The listing builds one solid part. Answer for the finished solid, in the listing's coordinates (mm). A direction names the side the tool comes from. Round coordinates to 2 decimals unless told otherwise and drop trailing zeros. Order: outer loops, then holes, each group sorted by start corner. A loop starts at its lowest first (then second) coordinate and runs counter-clockwise, first axis right, second up. Notation, with made-up numbers: (-29.5, 74) - (-6.5, 74) arc R6 cw to (-6.5, 84) - close; hole circle Ø7 at (-19.5, 35). An arc over 180 degrees is marked (long way). One line per item, written item: value. Start each with the question number.
1. For a pull along Y with two mould halves and no side action, classify faces 5 (the flat face through (-60, -9.941, 57)), 6 (the flat face through (-72.639, -2, -16)), 7 (the flat face through (-32, 19.559, -5)), 8 (the flat face through (-57, 5.559, -21)) as released by +Y, released by -Y, zero draft, split by the parting line, or undercut.
2. Section B-B, the plane x = -48 is taken. Give the vertices of the cut face in (y, z), then the cut area to 3 significant figures.
3. Section D-D, the plane x = -6.5 is taken. Give the vertices of the cut face in (y, z).
4. Section A-A, the plane z = -25 is taken. Give the vertices of the cut face in (x, y).
5. Flat-ended cylindrical pins translate along their axes: P1, Ø12, axis at x = 7.5, y = 18, coming from the -Z side; P2, Ø11, axis at x = -58.5, z = 88, coming from the -Y side; P3, Ø4, axis at y = 10, z = 30.5, coming from the +X side; P4, Ø11, axis at x = -58.5, z = 41, coming from the +Y side. Find the tip coordinate at first contact, or state that the pin passes through.
6. Straight lines are drawn through the part: line 1 (X direction, y = -0.5, z = -25); line 2 (Z direction, x = -21.5, y = 20); line 3 (X direction, y = -7, z = 59). For each, find the intervals that lie inside material, in ascending order.
7. A tool of negligible diameter and unlimited length cuts with its end or side. For faces 1 (the flat face through (-28.113, 13.002, -5.07)), 2 (the flat face through (-42.639, -2, -25)), 3 (the flat face through (-60, 4, 104.21)), 4 (the flat face through (-55.139, -9, 57)), from which of +Z, -Z, +X, -X, +Y, -Y can it reach the whole face along a straight path? Write none if from no direction.
8. Section C-C, the plane z = 96 is taken. Give the vertices of the cut face in (x, y).
from build123d import *

# Parameters (mm, degrees)
SKETCH3_W             = 42.5
SKETCH3_H             = 15
BOSS_EXTRUDE1_DEPTH   = 10
CUT_EXTRUDE1_DEPTH    = 2.5
SKETCH11_W            = 42.5
SKETCH11_H            = 10
BOSS_EXTRUDE5_DEPTH   = 10
SKETCH14_W            = 42.5
SKETCH14_H            = 10
BOSS_EXTRUDE7_DEPTH   = 15
SKETCH20_W            = 10
SKETCH20_H            = 40
BOSS_EXTRUDE10_DEPTH  = 50
SKETCH21_W            = 10
SKETCH21_H            = 25
BOSS_EXTRUDE11_DEPTH  = 113.5
SKETCH22_W            = 30
SKETCH22_H            = 6
BOSS_EXTRUDE12_DEPTH  = 30
SKETCH23_W            = 30
SKETCH23_H            = 30
BOSS_EXTRUDE13_DEPTH  = 8.5
FILLET1_R             = 3
CHAMFER1_SIZE         = 15
CHAMFER1_SIZE2        = 30.41699103
FILLET2_R             = 3
CHAMFER2_SIZE         = 10
CHAMFER2_SIZE2        = 17.320508076
FILLET3_R             = 5
CUT_EXTRUDE2_DEPTH    = 144.583262507
FILLET4_R             = 3
FILLET5_R             = 1.5
M8_TAPPED_HOLE1_D     = 6.8
M8_TAPPED_HOLE1_DEPTH = 22.25
M8_TAPPED_HOLE1_TIP   = 2.042926105
CUT_EXTRUDE3_DEPTH    = 141.312152004
FILLET6_R             = 1.5


with BuildPart() as part:
    # Sketch3 → Boss-Extrude1 (new body)
    with BuildSketch(Plane.XY):
        with Locations((-1.388845539, 0.05888455)):
            Rectangle(SKETCH3_W, SKETCH3_H)
    extrude(amount=-BOSS_EXTRUDE1_DEPTH)

    # Sketch2 → Cut-Extrude1 (cut)
    with BuildSketch(Plane.XY):
        with BuildLine():
            Line((-16.888114198, 2.469689731), (-3.968626967, 4.5))
            ThreePointArc((-3.968626967, 4.5), (0, 6), (3.968626967, 4.5))
            Line((3.968626967, 4.5), (16.888114198, 2.469689731))
            ThreePointArc((16.888114198, 2.469689731), (19, 0), (16.888114198, -2.469689731))
            Line((16.888114198, -2.469689731), (3.968626967, -4.5))
            ThreePointArc((3.968626967, -4.5), (0, -6), (-3.968626967, -4.5))
            Line((-3.968626967, -4.5), (-16.888114198, -2.469689731))
            ThreePointArc((-16.888114198, -2.469689731), (-19, 0), (-16.888114198, 2.469689731))
        make_face()
    extrude(amount=-CUT_EXTRUDE1_DEPTH, mode=Mode.SUBTRACT)

    # Sketch11 → Boss-Extrude5 (add)
    with BuildSketch(Plane.XZ.offset(7.44111545)):
        with Locations((-1.388845539, -5)):
            Rectangle(SKETCH11_W, SKETCH11_H)
    extrude(amount=BOSS_EXTRUDE5_DEPTH)

    # Sketch14 → Boss-Extrude7 (add)
    with BuildSketch(Plane(origin=(0, 7.55888455, 0), x_dir=(1, 0, 0), z_dir=(0, 1, 0))):
        with Locations((-1.388845539, 5)):
            Rectangle(SKETCH14_W, SKETCH14_H)
    extrude(amount=BOSS_EXTRUDE7_DEPTH)

    # Sketch20 → Boss-Extrude10 (add)
    with BuildSketch(Plane.ZY.offset(22.638845539)):
        with Locations((-5, 2.55888455)):
            Rectangle(SKETCH20_W, SKETCH20_H)
    extrude(amount=BOSS_EXTRUDE10_DEPTH)

    # Sketch21 → Boss-Extrude11 (add)
    with BuildSketch(Plane.XY):
        with Locations((-60.138845539, 2.55888455)):
            Rectangle(SKETCH21_W, SKETCH21_H)
    extrude(amount=BOSS_EXTRUDE11_DEPTH)

    # Sketch22 → Boss-Extrude12 (add)
    with BuildSketch(Plane(origin=(0, 0, -10), x_dir=(-1, 0, 0), z_dir=(0, 0, -1))):
        with Locations((57.638845539, 2.55888455)):
            Rectangle(SKETCH22_W, SKETCH22_H)
    extrude(amount=BOSS_EXTRUDE12_DEPTH)

    # Sketch23 → Boss-Extrude13 (add)
    with BuildSketch(Plane.XZ.offset(0.44111545)):
        with Locations((-57.638845539, -25)):
            Rectangle(SKETCH23_W, SKETCH23_H)
    extrude(amount=BOSS_EXTRUDE13_DEPTH)

    # Fillet1
    fillet1_edges = [part.edges().sort_by_distance(p)[0] for p in [
        (-65.138845539, 2.55888455, 0),
        (-60.138845539, -9.94111545, 0),
        (-55.138845539, 2.55888455, 0),
        (-60.138845539, 15.05888455, 0),
    ]]
    fillet(fillet1_edges, radius=FILLET1_R)

    # Chamfer1
    chamfer1_edges = [part.edges().sort_by_distance(p)[0] for p in [
        (19.861154461, 22.55888455, -5),
    ]]
    chamfer1_side = [part.faces().sort_by_distance(p)[0] for p in [
        (19.861154461, 2.55888455, -5),
    ]]
    chamfer(chamfer1_edges, length=CHAMFER1_SIZE, length2=CHAMFER1_SIZE2, reference=chamfer1_side[0])

    # Fillet2
    fillet2_edges = [part.edges().sort_by_distance(p)[0] for p in [
        (-10.555836569, 22.55888455, -5),
        (19.861154461, 7.55888455, -5),
    ]]
    fillet(fillet2_edges, radius=FILLET2_R)

    # Chamfer2
    chamfer2_edges = [part.edges().sort_by_distance(p)[0] for p in [
        (19.861154461, -17.44111545, -5),
    ]]
    chamfer2_side = [part.faces().sort_by_distance(p)[0] for p in [
        (19.861154461, -5.873875391, -5),
    ]]
    chamfer(chamfer2_edges, length=CHAMFER2_SIZE, length2=CHAMFER2_SIZE2, reference=chamfer2_side[0])

    # Fillet3
    fillet3_edges = [part.edges().sort_by_distance(p)[0] for p in [
        (2.540646385, -17.44111545, -5),
        (19.861154461, -7.44111545, -5),
    ]]
    fillet(fillet3_edges, radius=FILLET3_R)

    # Sketch24 → Cut-Extrude2 (cut, through all)
    with BuildSketch(Plane.ZY.offset(65.138845539)):
        Polygon((58.25, -6.94111545), (95.25, -6.94111545), (58.25, 12.05888455), (21.25, -6.94111545), align=None)
        Polygon((48.39896268, 12.05888455), (12.290027833, -6.483541453), (12.290027833, 12.05888455), align=None)
        Polygon((68.10103732, 12.05888455), (104.209972167, 12.05888455), (104.209972167, -6.483541453), align=None)
    extrude(amount=-CUT_EXTRUDE2_DEPTH, mode=Mode.SUBTRACT)

    # Fillet4
    fillet4_edges = [part.edges().sort_by_distance(p)[0] for p in [
        (-60.138845539, -6.483541453, 104.209972167),
        (-60.138845539, 12.05888455, 104.209972167),
        (-60.138845539, 12.05888455, 12.290027833),
        (-60.138845539, -6.483541453, 12.290027833),
        (-60.138845539, 12.05888455, 58.25),
    ]]
    fillet(fillet4_edges, radius=FILLET4_R)

    # Fillet5
    fillet5_edges = [part.edges().sort_by_distance(p)[0] for p in [
        (-60.138845539, 12.05888455, 68.10103732),
        (-60.138845539, 12.05888455, 48.39896268),
        (-60.138845539, -6.94111545, 21.25),
        (-60.138845539, -6.94111545, 95.25),
    ]]
    fillet(fillet5_edges, radius=FILLET5_R)

    # M8 Tapped Hole1
    with Locations(Plane(origin=(0, 5.55888455, 0), x_dir=(1, 0, 0), z_dir=(0, 1, 0))):
        with Locations((-57.638845539, 25)):
            Hole(M8_TAPPED_HOLE1_D / 2, depth=M8_TAPPED_HOLE1_DEPTH)
            with Locations((0, 0, -(M8_TAPPED_HOLE1_DEPTH + M8_TAPPED_HOLE1_TIP / 2))):  # 118° drill point
                Cone(0, M8_TAPPED_HOLE1_D / 2, M8_TAPPED_HOLE1_TIP, mode=Mode.SUBTRACT)

    # Sketch32 → Cut-Extrude3 (cut, through all)
    with BuildSketch(Plane(origin=(-42.638845539, 5.55888455, -10), x_dir=(1, 0, 0), z_dir=(0, 0, 1))):
        Polygon((10.809559843, 14), (3.309559843, 14), (10.809559843, 1.002474929), (18.309559843, 14), align=None)
        Polygon((1, 12), (9.65549398, -3), (1, -18), (1, -3), align=None)
        Polygon((10.809559843, -7.002474929), (18.309559843, -20), (10.809559843, -20), (3.309559843, -20), align=None)
        Polygon((20.619119687, -18), (20.619119687, -3), (20.619119687, 12), (11.963625707, -3), align=None)
    extrude(amount=CUT_EXTRUDE3_DEPTH, mode=Mode.SUBTRACT)

    # Fillet6
    fillet6_edges = [part.edges().sort_by_distance(p)[0] for p in [
        (-41.638845539, 17.55888455, -5),
        (-41.638845539, -12.44111545, -5),
        (-32.98335156, 2.55888455, -5),
        (-22.019725852, 17.55888455, -5),
        (-30.675219832, 2.55888455, -5),
        (-22.019725852, -12.44111545, -5),
        (-24.329285696, -14.44111545, -5),
        (-31.829285696, -1.44359038, -5),
        (-39.329285696, -14.44111545, -5),
        (-24.329285696, 19.55888455, -5),
        (-39.329285696, 19.55888455, -5),
        (-31.829285696, 6.561359479, -5),
    ]]
    fillet(fillet6_edges, radius=FILLET6_R)


solid = part.part
Answer list:
1. face 5: released by -Y
1. face 6: zero draft
1. face 7: undercut
1. face 8: released by +Y
2. outline: (-17.44, -10) - (-8.94, -10) - (-8.94, -40) - (5.56, -40) - (5.56, -10) - (22.56, -10) - (22.56, 0) - (-17.44, 0) - close
2. area: 835 mm²
3. outline: (-17.44, -10) - (20.56, -10) - (20.56, 0) - (4.1, 0) - (4.1, -2.5) - (-4.1, -2.5) - (-4.1, 0) - (-17.44, 0) - close
4. outline: (-72.64, -8.94) - (-61.04, -8.94) - (-61.04, 5.56) - (-72.64, 5.56) - close; (-54.24, -8.94) - (-42.64, -8.94) - (-42.64, 5.56) - (-54.24, 5.56) - close
5. P1: stops at z = -10
5. P2: stops at y = -9.94
5. P3: passes through
5. P4: stops at y = 15.06
6. line 1: x = -72.64 to -61.04, -54.24 to -42.64
6. line 2: z = -10 to 0
6. line 3: x = -65.14 to -55.14
7. face 1: +Z, -Z
7. face 2: -Z, +X, +Y, -Y
7. face 3: +X, -X
7. face 4: +Z, +X, +Y, -Y
8. outline: (-65.14, -9.94) - (-55.14, -9.94) - (-55.14, -2.27) - (-65.14, -2.27) - close; (-65.14, 12.06) - (-55.14, 12.06) - (-55.14, 15.06) - (-65.14, 15.06) - close
